```python
from build123d import *

# Parameters (mm, degrees)
SKETCH1_R           = 50
BOSS_EXTRUDE1_DEPTH = 50
BOSS_EXTRUDE2_REACH = 202
SKETCH2_R           = 45


with BuildPart() as part:
    # Sketch1 → Boss-Extrude1 (new body, symmetric)
    with BuildSketch(Plane.XY):
        with BuildLine():
            Line((-80, -40), (-80, 40))
            Line((-80, 40), (-25.912164589, 59.611741514))
            ThreePointArc((-25.912164589, 59.611741514), (64.980188395, 1.604716841), (-22.938091494, -60.818121959))
            Line((-22.938091494, -60.818121959), (-80, -40))
        make_face()
        Circle(SKETCH1_R, mode=Mode.SUBTRACT)
    extrude(amount=BOSS_EXTRUDE1_DEPTH, both=True)

    # Sketch2 → Boss-Extrude2 (add, up to next)
    with BuildSketch(Plane(origin=(120, 0, 0), x_dir=(0, 0, -1), z_dir=(1, 0, 0)), mode=Mode.PRIVATE) as boss_extrude2_sk1:
        Circle(SKETCH2_R)
    boss_extrude2_tool1 = extrude(boss_extrude2_sk1.sketch, amount=-BOSS_EXTRUDE2_REACH, mode=Mode.PRIVATE) - part.part
    add(boss_extrude2_tool1.solids().sort_by_distance((120, 0, 0))[0])

    # Sketch4 → Revolve2 (revolve)
    with BuildSketch(Plane(origin=(0, 0, 0), x_dir=(1, 0, 0), z_dir=(0, 1, 0))):
        Polygon((120, 0), (195, 0), (158.761034274, -7.465745985), (158.761034274, -12.083492049), (149, -14.256556682), (149, -25), (134, -25), (134, -20), (120, -20), align=None)
    revolve(axis=Axis((0, 0, 0), (1, 0, 0)))


solid = part.part
```
Build history of the part. All positions in model axes, mm. A direction names the side the tool comes from. Round coordinates to 2 decimals unless told otherwise and drop trailing zeros. Write each loop counter-clockwise with the first axis right and the second up, starting at its lowest first coordinate (ties: lowest second). Pieces come first, ordered by that corner, then holes.
1) Band-saw the part on C-C, the plane x = 0. List the corners of the cut face in (y, z), and give its area (3 significant figures).
2) 3-axis set-ups, long thin cutter, end or side, ignore diameter. For faces 1 (the flat face through (-51.07, -50.555, 0.7)), 2 (the cylindrical face through (126.902, 19.524, -4.336)), 3 (the cylindrical face through (141.395, -7.509, 23.846)): which of +Z, -Z, +X, -X, +Y, -Y reach the whole face in a straight line?
3) Band-saw the part on A-A, the plane x = 41. List the corners of the cut face in (y, z), and give its area (3 significant figures).
4) Band-saw the part on D-D, the plane z = 40. List the corners of the cut face in (x, y), and give its area (3 significant figures).
5) Pin check, flat tips, straight feed: pin 1 (12 mm diameter, centred on x = -25.5, z = -37.5, fed in from +Y); pin 2 (6 mm diameter, centred on x = -13, z = 8, fed in from +Y); pin 3 (8 mm diameter, centred on x = 100.5, z = -18.5, fed in from +Y); pin 4 (15 mm diameter, centred on y = -2.5, z = -2.5, fed in from +X). Stop position of each tip, or through.
6) Band-saw the part on B-B, the plane z = -36. List the corners of the cut face in (x, y), and give its area (3 significant figures).
7) Drill centre lines: probe 1 along Y at (x, z) = (0, -25); probe 2 along Y at (x, z) = (-7, 44.5); probe 3 along X at (y, z) = (9.5, -27.5). Where is each one in solid material? Low to high.
8) Mould opens along X. For faces 4 (the cylindrical face through (84, -27, 36)), 5 (the conical face through (176.63, -1.14, 3.61)), 6 (the flat face through (-80, -1, 1)), 7 (the flat face through (134, -17, -11)) say: +X half, -X half, draft (parallel to the pull), parting line (faces both ways), or undercut.
Ans:
1. outline: (-65, -50) - (-50, -50) - (-50, 50) - (-65, 50) - close; (50, -50) - (65, -50) - (65, 50) - (50, 50) - close
1. area: 3,000 mm2
2. face 1: +Z, -Z, -X, -Y
2. face 2: none
2. face 3: +X
3. outline: (-50.44, -50) - (-28.62, -50) - (-28.62, 50) - (-50.44, 50) - close; (28.62, -50) - (50.44, -50) - (50.44, 50) - (28.62, 50) - close
3. area: 4,360 mm2
4. outline: (-80, -40) - (-22.94, -60.82) arc R65 ccw to (61.64, -20.62) - (120, -20.62) - (120, 20.62) - (61.64, 20.62) arc R65 ccw to (-25.91, 59.61) - (-80, 40) - close; hole circle Ø100 at (0, 0)
4. area: 9,760 mm2
5. pin 1: stops at y = 62.01
5. pin 2: stops at y = 64.23
5. pin 3: stops at y = 42.6
5. pin 4: stops at x = 195
6. outline: (-80, -40) - (-22.94, -60.82) arc R65 ccw to (59.13, -27) - (120, -27) - (120, 27) - (59.13, 27) arc R65 ccw to (-25.91, 59.61) - (-80, 40) - close; hole circle Ø100 at (0, 0)
6. area: 10,500 mm2
7. probe 1: y = -65 to -50, 50 to 65
7. probe 2: y = -64.62 to -49.51, 49.51 to 64.62
7. probe 3: x = -80 to -49.09, 49.09 to 120
8. face 4: draft
8. face 5: +X half
8. face 6: -X half
8. face 7: undercut
